Build history of the part. All positions in model axes, mm. Face numbers are marked on the shaded views. A direction names the side the tool comes from. Give positions to 0.01 mm unless a question says otherwise; leave off trailing zeros. Write each loop counter-clockwise with the first axis right and the second up, starting at its lowest first coordinate (ties: lowest second). Pieces come first, ordered by that corner, then holes. Notation, with made-up numbers: M 73.25,69.25 L 117.25,69.25 A5 cw 117.25,75.25 Z; hole C 88,-6 d7. An arc over 180 degrees is marked long. One line per item, written item: value. Start each with the question number.
from build123d import *

# Parameters (mm, degrees)
SKETCH1_R           = 20.5
BOSS_EXTRUDE1_DEPTH = 2
SKETCH2_R           = 5.15
CUT_EXTRUDE1_DEPTH  = 3
SKETCH3_R           = 2
CUT_EXTRUDE2_DEPTH  = 2
BOSS_EXTRUDE4_DEPTH = 20


with BuildPart() as part:
    # Sketch1 → Boss-Extrude1 (new body)
    with BuildSketch(Plane(origin=(0, 0, 0), x_dir=(1, 0, 0), z_dir=(0, 1, 0))):
        with Locations(Location((0, 0, 0), (0, 0, 270))):
            Circle(SKETCH1_R)
    extrude(amount=BOSS_EXTRUDE1_DEPTH)

    # Sketch2 → Cut-Extrude1 (cut)
    with BuildSketch(Plane(origin=(0, 2, 0), x_dir=(1, 0, 0), z_dir=(0, 1, 0))):
        with Locations(Location((0, 0, 0), (0, 0, 270))):
            Circle(SKETCH2_R)
    extrude(amount=-CUT_EXTRUDE1_DEPTH, mode=Mode.SUBTRACT)

    # Sketch3 → Cut-Extrude2 (cut)
    with BuildSketch(Plane(origin=(0, 2, 0), x_dir=(1, 0, 0), z_dir=(0, 1, 0))):
        with Locations(Location((0, 16, 0), (0, 0, 270))):
            Circle(SKETCH3_R)
    extrude(amount=-CUT_EXTRUDE2_DEPTH, mode=Mode.SUBTRACT)

    # Sketch4 → Boss-Extrude4 (add)
    with BuildSketch(Plane(origin=(0, 2, 0), x_dir=(1, 0, 0), z_dir=(0, 1, 0))):
        with BuildLine():
            Line((-2.014609667, 7.214480564), (-11.484686708, 16.980929633))
            ThreePointArc((-11.484686708, 16.980929633), (-8.505321904, 18.650308428), (-5.290322683, 19.802358863))
            Line((-5.290322683, 19.802358863), (-5.290322683, 16))
            ThreePointArc((-5.290322683, 16), (0, 10.709677317), (5.290322683, 16))
            Line((5.290322683, 16), (5.290322683, 19.802019217))
            ThreePointArc((5.290322683, 19.802019217), (9.053928633, 18.389935215), (12.469975936, 16.271130881))
            Line((12.469975936, 16.271130881), (2.613547676, 7.214480564))
            ThreePointArc((2.613547676, 7.214480564), (0.299469005, 6.887955487), (-2.014609667, 7.214480564))
        make_face()
    extrude(amount=BOSS_EXTRUDE4_DEPTH)


solid = part.part
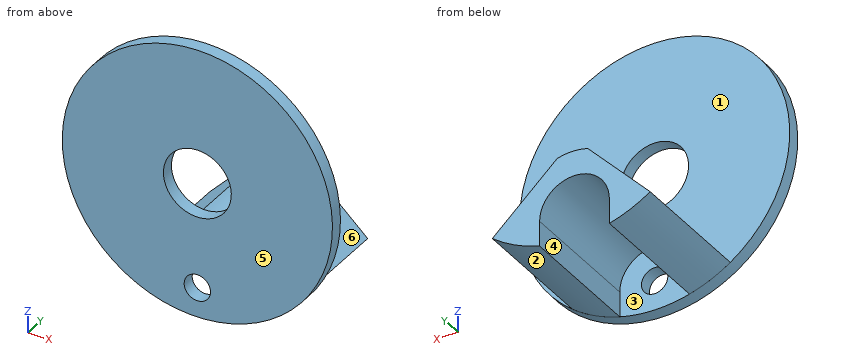
1) Drop flat-ended pins along their axis: P1, Ø1.9, axis at y = 11, z = -17, coming from the +X side; P2, Ø8, axis at y = 6.5, z = -9.5, coming from the +X side; P3, Ø8, axis at y = 4.5, z = 13, coming from the -X side. Give the stop position or say it passes through.
2) Band-saw the part on A-A (z = 0). List the corners of the cut face in (x, y), then the cut area to 3 significant figures.
3) Mould opens along X. For the marked faces 1, 2 and 3 say: released by +X, released by -X, zero draft, split by the parting line, or undercut.
4) Band-saw the part on B-B (x = 0). List the corners of the cut face in (y, z), then the cut area to 3 significant figures.
5) Band-saw the part on C-C (y = 19). List the corners of the cut face in (x, z), then the cut area to 3 significant figures.
6) Probe line 1 along X through (y, z) = (1.2, 0); line 2 along Y through (x, z) = (12.5, 10); line 3 along X through (y, z) = (0.55, -16). List the from-to ranges inside material, lowest first. Write a range as from..to.
7) Tool access for the marked faces 4, 5 and 6: list every direction of +Z, -Z, +X, -X, +Y, -Y with a clear straight run to the whole face (end or side of a thin tool).
8) Band-saw the part on D-D (x = 16). List the corners of the cut face in (y, z), then the cut area to 3 significant figures.
Model answer:
1. P1: stops at x = 12.47
1. P2: stops at x = 9.45
1. P3: stops at x = -17.96
2. outline: M -20.5,0 L -5.15,0 L -5.15,2 L -20.5,2 Z; M 5.15,0 L 20.5,0 L 20.5,2 L 5.15,2 Z
2. area: 61.4 mm²
3. face 1: zero draft
3. face 2: released by +X
3. face 3: undercut
4. outline: M 0,-20.5 L 2,-20.5 L 2,-18 L 0,-18 Z; M 0,-14 L 2,-14 L 2,-10.71 L 22,-10.71 L 22,-6.89 L 2,-6.89 L 2,-5.15 L 0,-5.15 Z; M 0,5.15 L 2,5.15 L 2,20.5 L 0,20.5 Z
4. area: 130 mm²
5. outline: M -11.48,-16.98 A20.52 ccw -5.29,-19.8 L -5.29,-16 A5.29 cw 5.29,-16 L 5.29,-19.8 A20.52 ccw 12.47,-16.27 L 2.61,-7.21 A8.36 ccw -2.01,-7.21 Z
5. area: 109 mm²
6. line 1: x = -20.5..-5.15, 5.15..20.5
6. line 2: y = 0..2
6. line 3: x = -12.82..-2, 2..12.82
7. face 4: -Z, +Y
7. face 5: +Z, -Z, +X, -X, -Y
7. face 6: +Z, +X, +Y
8. outline: M 0,-12.82 L 2,-12.82 L 2,12.82 L 0,12.82 Z
8. area: 51.3 mm²
